from build123d import *

# Parameters (mm, degrees)
PAD001_DEPTH    = 9.45
CHAMFER001_SIZE = 0.5
SKETCH003_R     = 1.25
HOLE_DEPTH      = 4.4
HOLE_TIPS_R     = 1.25


with BuildPart() as part:
    # ShapeBinder → Pad001 (new body, symmetric)
    with BuildSketch(Plane(origin=(0, 0, 4), x_dir=(1, 0, 0), z_dir=(0, 1, 0))):
        Polygon((-4.5, 4), (-10, 4), (-10, -4), (-4, -4), (-4, -3.55), (4, -3.55), (4, -4), (10, -4), (10, 4), (4.5, 4), (4.5, -0.5), (-4.5, -0.5), align=None)
    extrude(amount=PAD001_DEPTH, both=True)

    # Chamfer001
    chamfer001_edges = [part.edges().sort_by_distance(p)[0] for p in [
        (-10, 0, 8),
        (10, 0, 8),
        (10, 0, 0),
        (-10, 0, 0),
    ]]
    chamfer(chamfer001_edges, length=CHAMFER001_SIZE)

    # Sketch003 (on Face18 of Chamfer001) → Hole (cut)
    with BuildSketch(Plane(origin=(0, 0, 8), x_dir=(-1, 0, 0), z_dir=(0, 0, 1))):
        with Locations((-7.5, 5)):
            Circle(SKETCH003_R)
        with Locations((7.5, 5)):
            Circle(SKETCH003_R)
        with Locations((-7.5, -5)):
            Circle(SKETCH003_R)
        with Locations((7.5, -5)):
            Circle(SKETCH003_R)
    extrude(amount=-HOLE_DEPTH, mode=Mode.SUBTRACT)

    # Hole tips → Hole tip 1 section 0
    with BuildSketch(Plane(origin=(0, 0, 3.6), x_dir=(-1, 0, 0), z_dir=(0, 0, 1)), mode=Mode.PRIVATE) as hole_tip_1_s0:
        with Locations((-7.5, 5)):
            Circle(HOLE_TIPS_R)
    loft([hole_tip_1_s0.sketch, Vertex(7.5, -5, 2.848924)], mode=Mode.SUBTRACT)

    # Hole tips → Hole tip 2 section 0
    with BuildSketch(Plane(origin=(0, 0, 3.6), x_dir=(-1, 0, 0), z_dir=(0, 0, 1)), mode=Mode.PRIVATE) as hole_tip_2_s0:
        with Locations((7.5, 5)):
            Circle(HOLE_TIPS_R)
    loft([hole_tip_2_s0.sketch, Vertex(-7.5, -5, 2.848924)], mode=Mode.SUBTRACT)

    # Hole tips → Hole tip 3 section 0
    with BuildSketch(Plane(origin=(0, 0, 3.6), x_dir=(-1, 0, 0), z_dir=(0, 0, 1)), mode=Mode.PRIVATE) as hole_tip_3_s0:
        with Locations((-7.5, -5)):
            Circle(HOLE_TIPS_R)
    loft([hole_tip_3_s0.sketch, Vertex(7.5, 5, 2.848924)], mode=Mode.SUBTRACT)

    # Hole tips → Hole tip 4 section 0
    with BuildSketch(Plane(origin=(0, 0, 3.6), x_dir=(-1, 0, 0), z_dir=(0, 0, 1)), mode=Mode.PRIVATE) as hole_tip_4_s0:
        with Locations((7.5, -5)):
            Circle(HOLE_TIPS_R)
    loft([hole_tip_4_s0.sketch, Vertex(-7.5, 5, 2.848924)], mode=Mode.SUBTRACT)


solid = part.part
Input: part model. Units: mm. Frame: model coordinates. A direction names the side the tool comes from. Coordinates: 2 decimals unless noted, no trailing zeros. Loops run counter-clockwise (first coordinate to the right, second up) from the corner with the lowest first, then second, coordinate; pieces in that order, holes last. Notation, with made-up numbers: (-7.5, 80) -> (15.5, 80) arc R20 ccw to (15.5, 101) -> close; hole circle Ø9 at (51.25, -36.75). An arc over 180 degrees is marked (long way). Write item = value, one per line. Start each with the question number.
Item 1: Cut plane C-C, the plane x = -1.25. Return loops of the section in (y, z), plus the area to 3 significant figures.
Item 2: Cut plane B-B, the plane y = 7.5. Return loops of the section in (x, z), plus the area to 3 significant figures.
Item 3: Reachability of faces 1 (the face through (-4.5, 0, 2)), 2 (the face through (-6.51, 5.76, 5.83)), 3 (the face through (0, 0, 7.55)), 4 (the face through (10, 0, 4)), 5 (the face through (7, 0, 8)) from +Z, -Z, +X, -X, +Y, -Y: full face, straight path, thin tool, end or side. Return the list, or none.
Item 4: First-contact query: P1, Ø4.5, axis at x = 0.5, y = 0, coming from the -Z side; P2, Ø4, axis at x = -7.5, y = -5, coming from the +Z side; P3, Ø6.5, axis at x = -0.5, y = 1, coming from the +Z side. Flat tips, straight axial feed; report the tip coordinate or a pass-through.
Item 5: Material intervals for line 1 (Y direction, x = -7.5, z = 6.6); line 2 (X direction, y = 5, z = 6.3); line 3 (X direction, y = -3.25, z = 1.5), sorted ascending.
Item 6: Cut plane A-A, the plane z = 6.5. Return loops of the section in (x, y).
Item 7: Mould query, pull axis Y, two halves, no side actions, for faces 6 (the face through (7.66, 5.12, 2.97)), 7 (the face through (-7, 0, 0)), 8 (the face through (0, -9.45, 5)). Classes: pulls with the +Y half, pulls with the -Y half, needs draft (parallel to the pull), parting line crosses it, or undercut.
Ans:
q1.outline = (-9.45, 4.5) -> (9.45, 4.5) -> (9.45, 7.55) -> (-9.45, 7.55) -> close
q1.area = 57.6 mm²
q2.outline = (-10, 0.5) -> (-9.5, 0) -> (-4.5, 0) -> (-4.5, 4.5) -> (4.5, 4.5) -> (4.5, 0) -> (9.5, 0) -> (10, 0.5) -> (10, 7.5) -> (9.5, 8) -> (4, 8) -> (4, 7.55) -> (-4, 7.55) -> (-4, 8) -> (-9.5, 8) -> (-10, 7.5) -> close
q2.area = 115 mm²
q3.face_1 = -Z, +Y, -Y
q3.face_2 = +Z
q3.face_3 = +Z, +Y, -Y
q3.face_4 = +Z, -Z, +X, +Y, -Y
q3.face_5 = +Z, +X, -X, +Y, -Y
q4.P1 = 4.5
q4.P2 = 8
q4.P3 = 7.55
q5.line_1 = -9.45 to -6.25, -3.75 to 3.75, 6.25 to 9.45
q5.line_2 = -10 to -8.75, -6.25 to 6.25, 8.75 to 10
q5.line_3 = -10 to -4.5, 4.5 to 10
q6.outline = (-10, -9.45) -> (10, -9.45) -> (10, 9.45) -> (-10, 9.45) -> close; hole circle Ø2.5 at (-7.5, -5); hole circle Ø2.5 at (-7.5, 5); hole circle Ø2.5 at (7.5, -5); hole circle Ø2.5 at (7.5, 5)
q7.face_6 = undercut
q7.face_7 = needs draft
q7.face_8 = pulls with the -Y half
